Geometry check sheet. Reference: the model listing, model coordinates, mm. A direction names the side the tool comes from. Round coordinates to 2 decimals unless told otherwise and drop trailing zeros. Order: outer loops, then holes, each group sorted by start corner. A loop starts at its lowest first (then second) coordinate and runs counter-clockwise, first axis right, second up.
```python
from build123d import *

# Parameters (mm, degrees)
SKETCH1_W           = 1.5875
SKETCH1_H           = 31.75
BOSS_EXTRUDE1_DEPTH = 1.5875


with BuildPart() as part:
    # Sketch1 → Boss-Extrude1 (new body)
    # profile 1 of 3: a face of its own
    with BuildSketch(Plane(origin=(0, 0, 0), x_dir=(1, 0, 0), z_dir=(0, 1, 0))):
        with BuildLine():
            Line((11.1125, -39.6875), (11.1125, -15.875))
            Line((11.1125, -15.875), (11.1125, 15.875))
            Line((11.1125, 15.875), (11.1125, 39.6875))
            ThreePointArc((11.1125, 39.6875), (0, 31.259108818), (-11.1125, 39.6875))
            Line((-11.1125, 39.6875), (-11.1125, 15.875))
            Line((-11.1125, 15.875), (-11.1125, -15.875))
            Line((-11.1125, -15.875), (-11.1125, -39.6875))
            ThreePointArc((-11.1125, -39.6875), (0, -31.259108818), (11.1125, -39.6875))
        make_face()
        with BuildLine():
            ThreePointArc((-6.35, 20.146608818), (0, 26.496608818), (6.35, 20.146608818))
            Line((6.35, 20.146608818), (6.35, -20.146608818))
            ThreePointArc((6.35, -20.146608818), (0, -26.496608818), (-6.35, -20.146608818))
            Line((-6.35, -20.146608818), (-6.35, 20.146608818))
        make_face(mode=Mode.SUBTRACT)
    # profile 2 of 3: a face of its own
    with BuildSketch(Plane(origin=(0, 0, 0), x_dir=(1, 0, 0), z_dir=(0, 1, 0))):
        with Locations((-11.90625, 0)):
            Rectangle(SKETCH1_W, SKETCH1_H)
    # profile 3 of 3: a face of its own
    with BuildSketch(Plane(origin=(0, 0, 0), x_dir=(1, 0, 0), z_dir=(0, 1, 0))):
        with Locations((11.90625, 0)):
            Rectangle(SKETCH1_W, SKETCH1_H)
    extrude(amount=BOSS_EXTRUDE1_DEPTH)


solid = part.part
```
(1) Sectioned sample at A-A, the plane x = 0. Record the cut outline in (y, z), and give its area (3 significant figures).
Returned:
outline: (0, -31.26) - (1.59, -31.26) - (1.59, -26.5) - (0, -26.5) - close; (0, 26.5) - (1.59, 26.5) - (1.59, 31.26) - (0, 31.26) - close
area: 15.1 mm2
(2) Depth check by flat-ended pin: P1, Ø0.5, axis at x = 11.5, y = 1, coming from the -Z side (3 decimals); P2, Ø0.5, axis at y = 0.5, z = -33, coming from the -X side; P3, Ø0.5, axis at x = 12, y = 0.5, coming from the +Z side (3 decimals). Enter the tip coordinate at first touch or a pass-through.
Returned:
P1: stops at z = -15.875
P2: stops at x = -11.11
P3: stops at z = 15.875
(3) Set-up check for faces 1 (the flat face through (6.35, 1, 0)), 2 (the flat face through (-11.112, 1, 28)), 3 (the flat face through (12, 1, 15.875)), 4 (the flat face through (-11.112, 1, -28)), 5 (the flat face through (12, 1, -15.875)): record each of +Z, -Z, +X, -X, +Y, -Y from which the full face is reachable in a straight line by a thin tool's end or side.
Returned:
face 1: +Y, -Y
face 2: +Z, -X, +Y, -Y
face 3: +Z, +X, +Y, -Y
face 4: -Z, -X, +Y, -Y
face 5: -Z, +X, +Y, -Y
(4) Sectioned sample at D-D, the plane x = -9.75. Record the cut outline in (y, z), and give its area (3 significant figures).
Returned:
outline: (0, -36.63) - (1.59, -36.63) - (1.59, 36.63) - (0, 36.63) - close
area: 116 mm2
(5) Sectioned sample at B-B, the plane z = 10.5. Record the cut outline in (x, y), and give its area (3 significant figures).
Returned:
outline: (-12.7, 0) - (-6.35, 0) - (-6.35, 1.59) - (-12.7, 1.59) - close; (6.35, 0) - (12.7, 0) - (12.7, 1.59) - (6.35, 1.59) - close
area: 20.2 mm2
(6) Material ranges on line 1 (X direction, y = 0.7, z = 11.5); line 2 (X direction, y = 0.9, z = 17.5); line 3 (Z direction, x = 0.25, y = 0.1), recorded low to high.
Returned:
line 1: x = -12.7 to -6.35, 6.35 to 12.7
line 2: x = -11.11 to -6.35, 6.35 to 11.11
line 3: z = -31.26 to -26.49, 26.49 to 31.26
